```python
from build123d import *

# Parameters (mm, degrees)
SKIZZE2_R                            = 2.6
AUFSATZ_LINEAR_AUSTRAGEN1_DEPTH      = 10
SCHNITT_LINEAR_AUSTRAGEN1_DEPTH      = 44.890751019
SCHNITT_LINEAR_AUSTRAGEN1_DEPTH_BACK = 44.890751019
SKIZZE3_R                            = 1
SKIZZE3_W                            = 10
SKIZZE3_H                            = 22.630927951
SKIZZE4_W                            = 30
SKIZZE4_H                            = 13.4
SCHNITT_LINEAR_AUSTRAGEN2_DEPTH      = 44.890751019
SCHNITT_LINEAR_AUSTRAGEN3_DEPTH      = 44.890751019
SCHNITT_LINEAR_AUSTRAGEN3_DEPTH_BACK = 44.890751019
SKIZZE5_R                            = 2.7
SCHNITT_LINEAR_START                 = 15
SKIZZE6_R                            = 5
SCHNITT_LINEAR_AUSTRAGEN4_DEPTH      = 6
SCHNITT_LINEAR_START_2               = -15
SCHNITT_LINEAR_AUSTRAGEN5_DEPTH      = 6
AUFSATZ_LINEAR_START                 = -15
AUFSATZ_LINEAR_AUSTRAGEN2_DEPTH      = 10
SKIZZE10_R                           = 3
SCHNITT_LINEAR_AUSTRAGEN6_DEPTH      = 49.06659989
FASE1_SIZE                           = 4
VERRUNDUNG1_R                        = 10
VERRUNDUNG2_R                        = 10
SKIZZE11_R                           = 2.6
AUFSATZ_LINEAR_AUSTRAGEN3_DEPTH      = 7
VERRUNDUNG3_R                        = 4
SCHNITT_LINEAR_AUSTRAGEN7_DEPTH      = 3


with BuildPart() as part:
    # Skizze2 → Aufsatz-Linear austragen1 (new, symmetric)
    with BuildSketch(Plane(origin=(0, 0, 0), x_dir=(1, 0, 0), z_dir=(0, 1, 0))):
        Polygon((38, 13.445), (-38, 13.445), (-38, -1.555), (-15, -1.555), (-15, -19.555), (15, -19.555), (15, -1.555), (38, -1.555), align=None)
        with Locations(Location((-30, 5.945, 0), (0, 0, 270))):
            Circle(SKIZZE2_R, mode=Mode.SUBTRACT)
        with Locations(Location((30, 5.945, 0), (0, 0, 270))):
            Circle(SKIZZE2_R, mode=Mode.SUBTRACT)
        Polygon((0, -9.479978336), (7.212489168, -2.267489168), (0, 4.945), (-7.212489168, -2.267489168), align=None, mode=Mode.SUBTRACT)
    extrude(amount=AUFSATZ_LINEAR_AUSTRAGEN1_DEPTH, both=True)

    # Skizze3 → Schnitt-Linear austragen1 (cut, two sides: drawn at the far end of the back side and taken through both)
    with BuildSketch(Plane(origin=(0, 0, 0), x_dir=(1, 0, 0), z_dir=(0, 1, 0)).offset(-SCHNITT_LINEAR_AUSTRAGEN1_DEPTH_BACK)):
        with Locations((0, 4.945)):
            Circle(SKIZZE3_R)
        with Locations((-7.212489168, -2.267489168)):
            Circle(SKIZZE3_R)
        with Locations((7.212489168, -2.267489168)):
            Circle(SKIZZE3_R)
        with Locations((0, -15.795442312)):
            Rectangle(SKIZZE3_W, SKIZZE3_H)
    extrude(amount=SCHNITT_LINEAR_AUSTRAGEN1_DEPTH + SCHNITT_LINEAR_AUSTRAGEN1_DEPTH_BACK, mode=Mode.SUBTRACT)

    # Skizze4 → Schnitt-Linear austragen2 (cut, symmetric)
    with BuildSketch(Plane.XY):
        with Locations((30, 0)):
            Rectangle(SKIZZE4_W, SKIZZE4_H)
    schnitt_linear_austragen2 = extrude(amount=SCHNITT_LINEAR_AUSTRAGEN2_DEPTH, both=True, mode=Mode.SUBTRACT)

    # Spiegeln1: Schnitt-Linear austragen2 across plane
    add(schnitt_linear_austragen2.mirror(Plane(origin=(0, 0, 0), x_dir=(0, 0, 1), z_dir=(1, 0, 0))), mode=Mode.SUBTRACT)

    # Skizze5 → Schnitt-Linear austragen3 (cut, two sides: drawn at the far end of the back side and taken through both)
    with BuildSketch(Plane(origin=(0, 0, 0), x_dir=(0, 0, -1), z_dir=(1, 0, 0)).offset(-SCHNITT_LINEAR_AUSTRAGEN3_DEPTH_BACK)):
        with Locations((-12.855, 0)):
            Circle(SKIZZE5_R)
    extrude(amount=SCHNITT_LINEAR_AUSTRAGEN3_DEPTH + SCHNITT_LINEAR_AUSTRAGEN3_DEPTH_BACK, mode=Mode.SUBTRACT)

    # Skizze6 → Schnitt-Linear austragen4 (cut)
    with BuildSketch(Plane(origin=(0, 0, 0), x_dir=(0, 0, -1), z_dir=(1, 0, 0)).offset(SCHNITT_LINEAR_START)):
        with Locations((-12.855, 0)):
            Circle(SKIZZE6_R)
    extrude(amount=-SCHNITT_LINEAR_AUSTRAGEN4_DEPTH, mode=Mode.SUBTRACT)

    # Skizze7 → Schnitt-Linear austragen5 (cut)
    with BuildSketch(Plane(origin=(0, 0, 0), x_dir=(0, 0, -1), z_dir=(1, 0, 0)).offset(SCHNITT_LINEAR_START_2)):
        Polygon((-15.279871131, 4.2), (-17.704742261, 0), (-15.279871131, -4.2), (-10.430128869, -4.2), (-8.005257739, 0), (-10.430128869, 4.2), align=None)
    extrude(amount=SCHNITT_LINEAR_AUSTRAGEN5_DEPTH, mode=Mode.SUBTRACT)

    # Skizze9 → Aufsatz-Linear austragen2 (add)
    with BuildSketch(Plane(origin=(0, 0, 0), x_dir=(0, 0, -1), z_dir=(1, 0, 0)).offset(AUFSATZ_LINEAR_START)):
        Polygon((-1.555, -10), (13.445, -10), (0.445, -22), (-1.555, -22), align=None)
    aufsatz_linear_austragen2 = extrude(amount=-AUFSATZ_LINEAR_AUSTRAGEN2_DEPTH)

    # Spiegeln2: Aufsatz-Linear austragen2 across plane
    add(aufsatz_linear_austragen2.mirror(Plane.ZX))

    # Skizze10 → Schnitt-Linear austragen6 (cut, symmetric)
    with BuildSketch(Plane.XY):
        with Locations(Location((-20, -16, 0), (0, 0, 270))):
            Circle(SKIZZE10_R)
    schnitt_linear_austragen6 = extrude(amount=SCHNITT_LINEAR_AUSTRAGEN6_DEPTH, both=True, mode=Mode.SUBTRACT)

    # Spiegeln3: Schnitt-Linear austragen6 across plane
    add(schnitt_linear_austragen6.mirror(Plane.ZX), mode=Mode.SUBTRACT)

    # Fase1
    fase1_edges = [part.edges().sort_by_distance(p)[0] for p in [
        (-38, 8.35, -13.445),
        (-38, -8.35, -13.445),
        (38, 8.35, -13.445),
        (38, -8.35, -13.445),
    ]]
    chamfer(fase1_edges, length=FASE1_SIZE)

    # Verrundung1
    verrundung1_edges = [part.edges().sort_by_distance(p)[0] for p in [
        (38, 8.35, 1.555),
        (38, -8.35, 1.555),
        (-38, -8.35, 1.555),
        (-38, 8.35, 1.555),
    ]]
    fillet(verrundung1_edges, radius=VERRUNDUNG1_R)

    # Verrundung2
    verrundung2_edges = [part.edges().sort_by_distance(p)[0] for p in [
        (10, -10, 19.555),
        (-10, -10, 19.555),
        (-10, 10, 19.555),
        (10, 10, 19.555),
    ]]
    fillet(verrundung2_edges, radius=VERRUNDUNG2_R - 0.0001)  # a hair under: the kernel refuses the full size

    # Skizze11 → Aufsatz-Linear austragen3 (add)
    with BuildSketch(Plane(origin=(0, 0, -13.445), x_dir=(-1, 0, 0), z_dir=(0, 0, -1))):
        Polygon((10, -10), (15, -10), (15, -48), (-10, -48), (-10, -10), align=None)
        with Locations((-3, -41)):
            Circle(SKIZZE11_R, mode=Mode.SUBTRACT)
        with Locations((8, -35.8)):
            Circle(SKIZZE11_R, mode=Mode.SUBTRACT)
    extrude(amount=-AUFSATZ_LINEAR_AUSTRAGEN3_DEPTH)

    # Verrundung3
    verrundung3_edges = [part.edges().sort_by_distance(p)[0] for p in [
        (10, -48, -9.945),
        (-15, -48, -9.945),
    ]]
    fillet(verrundung3_edges, radius=VERRUNDUNG3_R)

    # Skizze12 → Schnitt-Linear austragen7 (cut)
    with BuildSketch(Plane.XY.offset(-6.445)):
        Polygon((5.424871131, -36.8), (0.575128869, -36.8), (-1.849742261, -41), (0.575128869, -45.2), (5.424871131, -45.2), (7.849742261, -41), align=None)
        Polygon((-10.424871131, -40), (-5.575128869, -40), (-3.150257739, -35.8), (-5.575128869, -31.6), (-10.424871131, -31.6), (-12.849742261, -35.8), align=None)
    extrude(amount=-SCHNITT_LINEAR_AUSTRAGEN7_DEPTH, mode=Mode.SUBTRACT)


solid = part.part
```
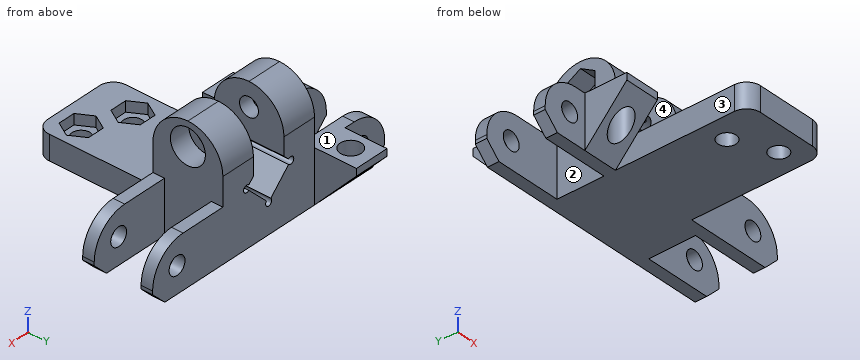
CAD build for the part. Positions are in the model's coordinates, mm. Face numbers are marked on the shaded views. A direction names the side the tool comes from. Give positions to 0.01 mm unless a question says otherwise; leave off trailing zeros. Order: outer loops, then holes, each group sorted by start corner. A loop starts at its lowest first (then second) coordinate and runs counter-clockwise, first axis right, second up.
(1) Saw through at A-A, the plane x = 25. Give the cut face in (y, z) (3 decimals).
(2) Saw through at C-C, the plane x = -30. Give the cut face in (y, z) (3 decimals).
(3) Flat gauge pins, fed straight in: pin 1 (6 mm diameter, centred on y = 4, z = -3.5, fed in from +X); pin 2 (4 mm diameter, centred on x = 19.5, z = -7.5, fed in from +Y); pin 3 (4.5 mm diameter, centred on x = -29, z = -7, fed in from -Y); pin 4 (1.2 mm diameter, centred on x = 0, z = -4.945, fed in from -Y). Where does each tip first touch, or does it go through?
(4) Saw through at D-D, the plane x = 2. Give the cut face in (y, z) (3 decimals), then the cut area to 3 significant figures.
(5) Drill centre lines: L1, parallel to Y at x = 33, z = -1.5; L2, parallel to Y at x = -8, z = -10.4; L3, parallel to Y at x = 9, z = 4. Where is each one in solid material? Low to high.
(6) Tool access for the marked faces 1, 2, 3 and 4: list every direction of +Z, -Z, +X, -X, +Y, -Y with a clear straight run to the whole face (end or side of a thin tool).
(7) Saw through at B-B, the plane y = 16. Give the cut face in (x, z) (3 decimals), then the cut area to 3 significant figures.
Results found:
1. outline: (-10, -13.445) - (-6.7, -13.445) - (-6.7, 1.555) - (-10, 1.555) - close; (6.7, -13.445) - (10, -13.445) - (10, 1.555) - (6.7, 1.555) - close
2. outline: (-10, -13.445) - (-6.7, -13.445) - (-6.7, -8.545) - (-10, -8.545) - close; (-10, -3.345) - (-6.7, -3.345) - (-6.7, 1.353) - (-10, 1.353) - close; (6.7, -13.445) - (10, -13.445) - (10, -8.545) - (6.7, -8.545) - close; (6.7, -3.345) - (10, -3.345) - (10, 1.353) - (6.7, 1.353) - close
3. pin 1: stops at x = 37.32
3. pin 2: stops at y = 10
3. pin 3: stops at y = -10
3. pin 4: passes through
4. outline: (-48, -13.445) - (-43.4, -13.445) - (-43.4, -9.445) - (-45.2, -9.445) - (-45.2, -6.445) - (-48, -6.445) - close; (-38.6, -13.445) - (10, -13.445) - (10, -2.945) - (-10, -2.945) - (-10, -6.445) - (-36.8, -6.445) - (-36.8, -9.445) - (-38.6, -9.445) - close
4. area: 432 mm2
5. L1: y = -10 to -6.7, 6.7 to 10
5. L2: y = -48 to -38.4, -33.2 to 10
5. L3: y = -10 to 10
6. face 1: +Z, -X, +Y, -Y
6. face 2: +Z, -X
6. face 3: -Z, -X, -Y
6. face 4: +Z, +Y, -Y
7. outline: (-25, -6.945) - (-23, -6.945) - (-23, 1.555) - (-25, 1.555) - close; (-17, -6.945) - (-15, -6.945) - (-15, 1.555) - (-17, 1.555) - close
7. area: 34.0 mm2
